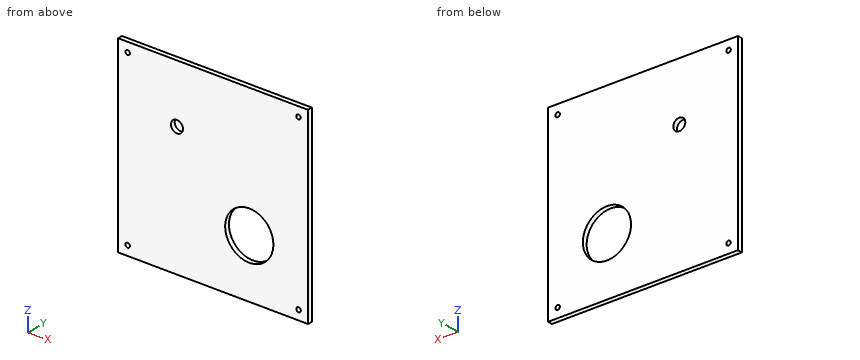
from build123d import *

# Parameters (mm, degrees)
SKETCH1_W           = 200
SKETCH1_H           = 200
BOSS_EXTRUDE1_DEPTH = 2.5
SKETCH2_R           = 2.38125
CUT_EXTRUDE1_DEPTH  = 5
SKETCH3_R           = 6.35
CUT_EXTRUDE2_DEPTH  = 5
SKETCH4_R           = 25.4
CUT_EXTRUDE3_DEPTH  = 142.509716981


with BuildPart() as part:
    # Sketch1 → Boss-Extrude1 (new, symmetric)
    with BuildSketch(Plane(origin=(0, 0, 0), x_dir=(1, 0, 0), z_dir=(0, 1, 0))):
        Rectangle(SKETCH1_W, SKETCH1_H)
    extrude(amount=BOSS_EXTRUDE1_DEPTH, both=True)

    # Sketch2 → Cut-Extrude1 (cut)
    with BuildSketch(Plane(origin=(0, 2.5, 0), x_dir=(1, 0, 0), z_dir=(0, 1, 0))):
        with Locations(Location((-90, 90, 0), (0, 0, 270))):
            Circle(SKETCH2_R)
        with Locations(Location((90, 90, 0), (0, 0, 270))):
            Circle(SKETCH2_R)
        with Locations(Location((-90, -90, 0), (0, 0, 270))):
            Circle(SKETCH2_R)
        with Locations(Location((90, -90, 0), (0, 0, 270))):
            Circle(SKETCH2_R)
    extrude(amount=-CUT_EXTRUDE1_DEPTH, mode=Mode.SUBTRACT)

    # Sketch3 → Cut-Extrude2 (cut)
    with BuildSketch(Plane(origin=(0, 2.5, 0), x_dir=(1, 0, 0), z_dir=(0, 1, 0))):
        with Locations(Location((-38.1, -38.1, 0), (0, 0, 270))):
            Circle(SKETCH3_R)
    extrude(amount=-CUT_EXTRUDE2_DEPTH, mode=Mode.SUBTRACT)

    # Sketch4 → Cut-Extrude3 (cut, through all)
    with BuildSketch(Plane(origin=(0, 2.5, 0), x_dir=(1, 0, 0), z_dir=(0, 1, 0))):
        with Locations(Location((38.1, 38.1, 0), (0, 0, 270))):
            Circle(SKETCH4_R)
    extrude(amount=-CUT_EXTRUDE3_DEPTH, mode=Mode.SUBTRACT)


solid = part.part
Source: CAD feature listing. Evaluate the final solid. Frame: model axes, mm. Give positions to 0.01 mm unless a question says otherwise; leave off trailing zeros. Write each loop counter-clockwise with the first axis right and the second up, starting at its lowest first coordinate (ties: lowest second). Pieces come first, ordered by that corner, then holes. Notation, with made-up numbers: M 9,-40 L 58,-40 A16 cw 58,-19 Z; hole C -29.75,-6.5 d9. An arc over 180 degrees is marked long. Return JSON: item names as keys, results as strings. Group by question number.
1) Cut plane D-D, the plane x = 90. Output: boundary loops of the cut face in (y, z).
2) Cut plane A-A, the plane x = -38.1. Output: boundary loops of the cut face in (y, z).
3) Ray query, L1, parallel to X at y = 0.45, z = 90; L2, parallel to X at y = 0.6, z = -38.1; L3, parallel to X at y = -0.55, z = 38.1. Return the intervals inside material, ascending.
4) First-contact query: pin 1 Ø5.5 at (x, z) = (90, 90) entering from +Y. Flat tip, straight axial feed; report the tip coordinate or a pass-through.
5) Cut plane B-B, the plane z = 38.1. Output: boundary loops of the cut face in (x, y).
6) Cut plane C-C, the plane y = 0.1. Output: boundary loops of the cut face in (x, z), then the cut area to 3 significant figures.
Data:
{
 "1": {"outline": "M -2.5,-100 L 2.5,-100 L 2.5,-92.38 L -2.5,-92.38 Z; M -2.5,-87.62 L 2.5,-87.62 L 2.5,87.62 L -2.5,87.62 Z; M -2.5,92.38 L 2.5,92.38 L 2.5,100 L -2.5,100 Z"},
 "2": {"outline": "M -2.5,-100 L 2.5,-100 L 2.5,31.75 L -2.5,31.75 Z; M -2.5,44.45 L 2.5,44.45 L 2.5,100 L -2.5,100 Z"},
 "3": {"L1": "x = -100 to -92.38, -87.62 to 87.62, 92.38 to 100", "L2": "x = -100 to 12.7, 63.5 to 100", "L3": "x = -100 to -44.45, -31.75 to 100"},
 "4": {"pin 1": "stops at y = 2.5"},
 "5": {"outline": "M -100,-2.5 L -44.45,-2.5 L -44.45,2.5 L -100,2.5 Z; M -31.75,-2.5 L 100,-2.5 L 100,2.5 L -31.75,2.5 Z"},
 "6": {"outline": "M -100,-100 L 100,-100 L 100,100 L -100,100 Z; hole C -90,-90 d4.76; hole C -90,90 d4.76; hole C -38.1,38.1 d12.7; hole C 38.1,-38.1 d50.8; hole C 90,-90 d4.76; hole C 90,90 d4.76", "area": "37,800 mm²"}
}
